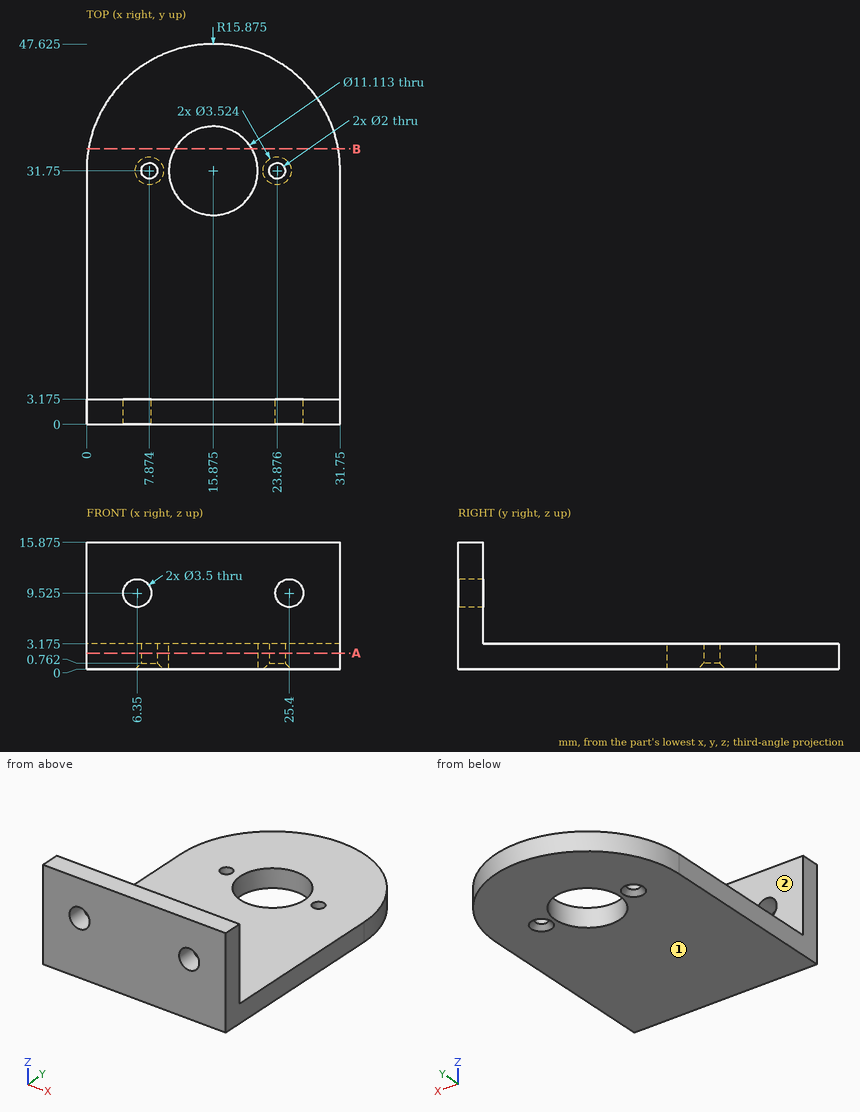
Print and shaded views of the part. All mm, measured from the part's lowest x, y and z. A direction names the side the tool comes from. Coordinates: 2 decimals unless noted, no trailing zeros. Loops run counter-clockwise (first coordinate to the right, second up) from the corner with the lowest first, then second, coordinate; pieces in that order, holes last. Notation, with made-up numbers: (60.25, 54.5) -> (84.25, 54.5) arc R26 ccw to (84.25, 85.5) -> close; hole circle Ø7 at (23.5, -11). An arc over 180 degrees is marked (long way). Use a Markdown table: item, result. Add a question column.
Item 1: Band-saw the part on B-B on y = 34.5. Write the cut outline in (x, z) (1 decimal).
Item 2: Which spindle directions (+Z, -Z, +X, -X, +Y, -Y) get a long thin tool onto all of the face, cutting with end or side? Do the marked faces 1 and 2. Say none if no direction does.
Item 3: Flat gauge pins, fed straight in: P1, Ø4.5, axis at x = 25.4, z = 9.525, coming from the +Y side (1 decimal); P2, Ø6, axis at x = 7, y = 40.5, coming from the +Z side (1 decimal); P3, Ø4, axis at x = 27.5, z = 2, coming from the +Y side (1 decimal). Where does each tip first touch, or does it go through?
Item 4: Band-saw the part on A-A on z = 2. Give the number of separate pieces and of enclosed holes in the cut face, plus the area to 3 significant figures.
Item 5: Probe probe 1 along Z at (x, y) = (9, 40) (1 decimal); probe 2 along Y at (x, z) = (10, 1.25). List the from-to ranges inside material, lowest first.
Geometry says:
| question | item | result |
|---|---|---|
| 1 | outline | (0.2, 0) -> (11, 0) -> (11, 3.2) -> (0.2, 3.2) -> close; (20.7, 0) -> (31.5, 0) -> (31.5, 3.2) -> (20.7, 3.2) -> close |
| 2 | face 1 | -Z, +X, -X, +Y, -Y |
| 2 | face 2 | +Z, +X, -X, +Y |
| 3 | P1 | y = 3.2 |
| 3 | P2 | z = 3.2 |
| 3 | P3 | y = 44.4 |
| 4 | separate pieces | 1 |
| 4 | enclosed holes | 3 |
| 4 | area | 1,300 mm² |
| 5 | probe 1 | 0 to 3.2 |
| 5 | probe 2 | 0 to 46.5 |
